```python
from build123d import *

# Parameters (mm, degrees)
SKETCH_W   = 488.95
SKETCH_H   = 501.65
SKETCH_W_2 = 387.35
SKETCH_H_2 = 400.05
PAD_DEPTH  = 6.35


with BuildPart() as part:
    # Sketch → Pad (new body)
    with BuildSketch(Plane.XZ):
        Rectangle(SKETCH_W, SKETCH_H)
        Rectangle(SKETCH_W_2, SKETCH_H_2, mode=Mode.SUBTRACT)
    extrude(amount=PAD_DEPTH)


solid = part.part
```
Check sheet for the modelled part. Datum: model origin and axes. Units: mm. Give positions to 0.01 mm unless a question says otherwise; leave off trailing zeros. Order: outer loops, then holes, each group sorted by start corner. A loop starts at its lowest first (then second) coordinate and runs counter-clockwise, first axis right, second up. Notation, with made-up numbers: M 72.25,5 L 115.25,5 A22 ccw 115.25,22 Z; hole C 36.5,6 d5. An arc over 180 degrees is marked long. Answer in a Markdown table with one row per item.
1) Cross-section at A-A, the plane x = -144.5. Enter the section's corners in (y, z) (3 decimals), plus the area to 3 significant figures.
Filled sheet:
| item | result |
|---|---|
| outline | M -6.35,-250.825 L 0,-250.825 L 0,-200.025 L -6.35,-200.025 Z; M -6.35,200.025 L 0,200.025 L 0,250.825 L -6.35,250.825 Z |
| area | 645 mm2 |
2) Gauge pin test, flat end, axial feed: P1, Ø12, axis at x = 152, z = 193.5, coming from the -Y side. Record the tip position at first contact, or that the pin passes through.
Filled sheet:
| item | result |
|---|---|
| P1 | passes through |
3) Thickness scan on L1, parallel to X at y = -3, z = 58 (3 decimals); L2, parallel to Z at x = -82.5, y = -0.25 (3 decimals). Record the ranges inside material, lowest first. Write a range as [from, to].
Filled sheet:
| item | result |
|---|---|
| L1 | x = [-244.475, -193.675], [193.675, 244.475] |
| L2 | z = [-250.825, -200.025], [200.025, 250.825] |
4) Cross-section at C-C, the plane z = 46. Enter the section's corners in (x, y) (3 decimals).
Filled sheet:
| item | result |
|---|---|
| outline | M -244.475,-6.35 L -193.675,-6.35 L -193.675,0 L -244.475,0 Z; M 193.675,-6.35 L 244.475,-6.35 L 244.475,0 L 193.675,0 Z |
5) Cross-section at B-B, the plane y = -4.5. Enter the section's corners in (x, z) (3 decimals), plus the area to 3 significant figures.
Filled sheet:
| item | result |
|---|---|
| outline | M -244.475,-250.825 L 244.475,-250.825 L 244.475,250.825 L -244.475,250.825 Z; hole M -193.675,-200.025 L 193.675,-200.025 L 193.675,200.025 L -193.675,200.025 Z |
| area | 90,300 mm2 |
